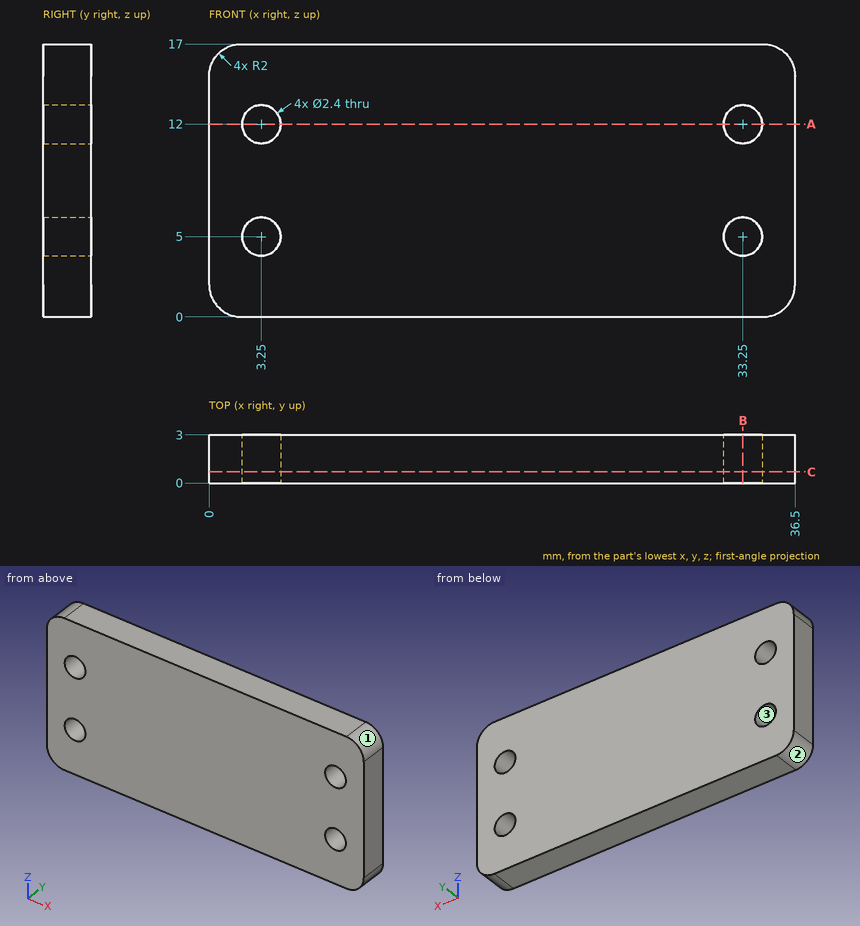
Design review of the part shown in the three views and the two pictorial views. Dimensions are in mm from the part's minimum x, y and z. Round coordinates to 2 decimals unless told otherwise and drop trailing zeros. Loops run counter-clockwise (first coordinate to the right, second up) from the corner with the lowest first, then second, coordinate; pieces in that order, holes last. Notation, with made-up numbers: (-6, -21.75) -> (20, -21.75) arc R19 cw to (20, -14.75) -> close; hole circle Ø6 at (24, 72). An arc over 180 degrees is marked (long way). Use one line per item in the form item = value. Start each with the question number.
Q1. We need section B-B on x = 33.25. Give the boundary of the cut face in (y, z), then the cut area to 3 significant figures.
Q2. For pin 1 Ø1.4 at (x, z) = (33.25, 12) entering from -Y, flat-tipped, find the tip position at first contact; note if it passes through.
Q3. Wall thickness on line 1 along Z through (x, y) = (3.25, 2.2); line 2 along X through (y, z) = (1.5, 5); line 3 along X through (y, z) = (1.05, 12.75): over which ranges is each line inside the solid? List them lowest first. Write a range as [from, to].
Q4. We need section C-C on y = 0.7. Give the boundary of the cut face in (x, z), then the cut area to 3 significant figures.
Q5. We need section A-A on z = 12. Give the boundary of the cut face in (x, y), then the cut area to 3 significant figures.
Q6. Draft analysis for pull direction X (two halves, no side actions). For the marked faces 1, 2 and 3, state which applies: +X half, -X half, draft (parallel to the pull), parting line (faces both ways), or undercut.
Calculated:
q1.outline = (0, 0) -> (3, 0) -> (3, 3.8) -> (0, 3.8) -> close; (0, 6.2) -> (3, 6.2) -> (3, 10.8) -> (0, 10.8) -> close; (0, 13.2) -> (3, 13.2) -> (3, 17) -> (0, 17) -> close
q1.area = 36.6 mm²
q2.pin_1 = through
q3.line_1 = [0, 3.8], [6.2, 10.8], [13.2, 17]
q3.line_2 = [0, 2.05], [4.45, 32.05], [34.45, 36.5]
q3.line_3 = [0, 2.31], [4.19, 32.31], [34.19, 36.5]
q4.outline = (0, 2) arc R2 ccw to (2, 0) -> (34.5, 0) arc R2 ccw to (36.5, 2) -> (36.5, 15) arc R2 ccw to (34.5, 17) -> (2, 17) arc R2 ccw to (0, 15) -> close; hole circle Ø2.4 at (3.25, 5); hole circle Ø2.4 at (3.25, 12); hole circle Ø2.4 at (33.25, 5); hole circle Ø2.4 at (33.25, 12)
q4.area = 599 mm²
q5.outline = (0, 0) -> (2.05, 0) -> (2.05, 3) -> (0, 3) -> close; (4.45, 0) -> (32.05, 0) -> (32.05, 3) -> (4.45, 3) -> close; (34.45, 0) -> (36.5, 0) -> (36.5, 3) -> (34.45, 3) -> close
q5.area = 95.1 mm²
q6.face_1 = +X half
q6.face_2 = -X half
q6.face_3 = undercut
